Source: CAD feature listing. Evaluate the final solid. Frame: model axes, mm. Face numbers are marked on the shaded views. Round coordinates to 2 decimals unless told otherwise and drop trailing zeros. Write each loop counter-clockwise with the first axis right and the second up, starting at its lowest first coordinate (ties: lowest second). Pieces come first, ordered by that corner, then holes. Notation, with made-up numbers: (74, 82.5) -> (104, 82.5) arc R13 cw to (104, 87.5) -> close; hole circle Ø7 at (-15.75, 84). An arc over 180 degrees is marked (long way). Return JSON: item names as keys, results as strings. Group by question number.
from build123d import *

# Parameters (mm, degrees)
F1_DEPTH = 3
F0_R     = 9.5
F0_R_2   = 5.5
F2_DEPTH = 4.5
F3_SIZE  = 1


with BuildPart() as f1:
    # F0 (on Front) → F1 (new body, symmetric)
    with BuildSketch(Plane.XZ):
        with BuildLine():
            ThreePointArc((13.333333, 90.09288), (0, 85), (-13.333333, 90.09288))
            ThreePointArc((-13.333333, 90.09288), (-10.871291, 86.721803), (-10, 82.63932))
            Line((-10, 82.63932), (-10, 15))
            ThreePointArc((-10, 15), (-10.513167, 11.837722), (-12, 9))
            ThreePointArc((-12, 9), (0, 15), (12, 9))
            ThreePointArc((12, 9), (10.513167, 11.837722), (10, 15))
            Line((10, 15), (10, 82.63932))
            ThreePointArc((10, 82.63932), (10.871291, 86.721803), (13.333333, 90.09288))
        make_face()
    extrude(amount=F1_DEPTH, both=True)

    # F0 (on Front) → F2 (join, symmetric)
    with BuildSketch(Plane.XZ):
        with BuildLine():
            ThreePointArc((13.333333, 90.09288), (18.257419, 96.835034), (20, 105))
            ThreePointArc((20, 105), (-8.164966, 123.257419), (-13.333333, 90.09288))
            ThreePointArc((-13.333333, 90.09288), (0, 85), (13.333333, 90.09288))
        make_face()
        with Locations((0, 105)):
            Circle(F0_R, mode=Mode.SUBTRACT)
        with BuildLine():
            ThreePointArc((12, 9), (0, 15), (-12, 9))
            ThreePointArc((-12, 9), (-4.743416, -14.230249), (15, 0))
            ThreePointArc((15, 0), (14.230249, 4.743416), (12, 9))
        make_face()
        Circle(F0_R_2, mode=Mode.SUBTRACT)
    extrude(amount=F2_DEPTH, both=True)

    # F3
    f3_edges = [f1.edges().sort_by_distance(p)[0] for p in [
        (18.257419, -4.5, 96.835034),
        (-8.164966, -4.5, 123.257419),
        (0, -4.5, 85),
        (-9.5, -4.5, 105),
        (14.230249, -4.5, 4.743416),
        (0, -4.5, 15),
        (-4.743416, -4.5, -14.230249),
        (-5.5, -4.5, 0),
        (-4.743416, 4.5, -14.230249),
        (-5.5, 4.5, 0),
        (18.257419, 4.5, 96.835034),
        (-8.164966, 4.5, 123.257419),
        (0, 4.5, 85),
        (-9.5, 4.5, 105),
    ]]
    chamfer(f3_edges, length=F3_SIZE)


solid = f1.part
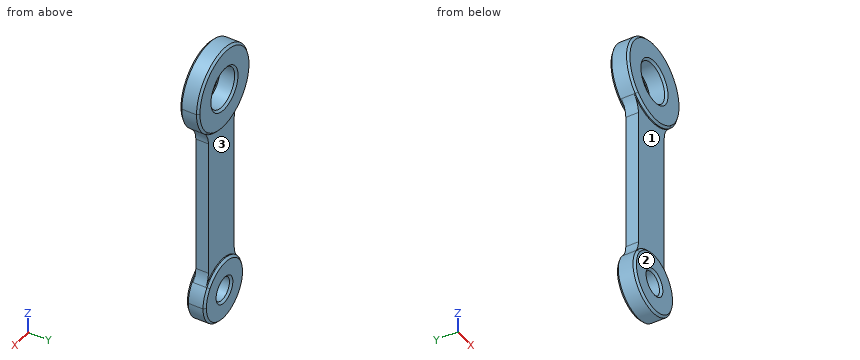
Item 1: Cut plane C-C on z = 64. Output: boundary loops of the cut face in (x, y), and give its area (3 significant figures).
Item 2: Cut plane A-A on y = -0.75. Output: boundary loops of the cut face in (x, z), and give its area (3 significant figures).
Item 3: Cut plane B-B on x = 0. Give the number of separate pieces and of enclosed holes in the cut face, and give its area (3 significant figures).
Item 4: Material intervals for probe 1 along Z at (x, y) = (0, -2); probe 2 along Z at (x, y) = (-4, -3.25); probe 3 along Z at (x, y) = (-2, 0.75), sorted ascending.
Item 5: First-contact query: pin 1 Ø13.5 at (x, z) = (-2.5, 60) entering from +Y; pin 2 Ø4 at (y, z) = (1, 92) entering from -X; pin 3 Ø3 at (y, z) = (-1, -0.5) entering from +X. Flat tips, straight axial feed; report the tip coordinate or a pass-through.
Item 6: Pull-direction query (Z, two-part tool) for the marked faces 1, 2 and 3; classes: +Z half, -Z half, draft (parallel to the pull), parting line (faces both ways), or undercut.
Here are the results:
{
 "1": {"outline": "(-10, -3) -> (10, -3) -> (10, 3) -> (-10, 3) -> close", "area": "120 mm^2"},
 "2": {"outline": "(-13.33, 90.09) arc R10 cw to (-10, 82.64) -> (-10, 15) arc R10 cw to (-12, 9) arc R15 ccw (long way) to (15, 0) arc R15 ccw to (12, 9) arc R10 cw to (10, 15) -> (10, 82.64) arc R10 cw to (13.33, 90.09) arc R20 ccw to (20, 105) arc R20 ccw (long way) to start; hole circle Ø19 at (0, 105); hole circle Ø11 at (0, 0)", "area": "3,040 mm^2"},
 "3": {"separate pieces": "3", "enclosed holes": "0", "area": "772 mm^2"},
 "4": {"probe 1": "z = -15 to -5.5, 5.5 to 95.5, 114.5 to 125", "probe 2": "z = -14.46 to -3.77, 3.77 to 14.46, 85.4 to 96.38, 113.62 to 124.6", "probe 3": "z = -14.87 to -5.12, 5.12 to 95.71, 114.29 to 124.9"},
 "5": {"pin 1": "stops at y = 3", "pin 2": "stops at x = -16.7", "pin 3": "stops at x = 15"},
 "6": {"face 1": "undercut", "face 2": "draft", "face 3": "undercut"}
}
